```python
from build123d import *

# Parameters (mm, degrees)
CROQUIS1_W              = 74.8
CROQUIS1_H              = 11.8
SALIENTE_EXTRUIR1_DEPTH = 2.5
CORTAR_EXTRUIR1_REACH   = 4.5
CROQUIS2_R              = 1.6


with BuildPart() as part:
    # Croquis1 → Saliente-Extruir1 (new body)
    with BuildSketch(Plane.XY):
        with Locations((0, -76)):
            Rectangle(CROQUIS1_W, CROQUIS1_H)
    extrude(amount=SALIENTE_EXTRUIR1_DEPTH)

    # Croquis2 → Cortar-Extruir1 (cut, up to next)
    with BuildSketch(Plane.XY.offset(2.5), mode=Mode.PRIVATE) as cortar_extruir1_sk1:
        with Locations((-22.5, -76)):
            Circle(CROQUIS2_R)
    cortar_extruir1_tool1 = extrude(cortar_extruir1_sk1.sketch, amount=-CORTAR_EXTRUIR1_REACH, mode=Mode.PRIVATE) & part.part
    add(cortar_extruir1_tool1.solids().sort_by_distance((-22.5, -76, 2.5))[0], mode=Mode.SUBTRACT)
    # Croquis2 → Cortar-Extruir1 (cut, up to next)
    with BuildSketch(Plane.XY.offset(2.5), mode=Mode.PRIVATE) as cortar_extruir1_sk2:
        with Locations((22.5, -76)):
            Circle(CROQUIS2_R)
    cortar_extruir1_tool2 = extrude(cortar_extruir1_sk2.sketch, amount=-CORTAR_EXTRUIR1_REACH, mode=Mode.PRIVATE) & part.part
    add(cortar_extruir1_tool2.solids().sort_by_distance((22.5, -76, 2.5))[0], mode=Mode.SUBTRACT)
    # Croquis2 → Cortar-Extruir1 (cut, up to next)
    with BuildSketch(Plane.XY.offset(2.5), mode=Mode.PRIVATE) as cortar_extruir1_sk3:
        with Locations((-7.5, -76)):
            Circle(CROQUIS2_R)
    cortar_extruir1_tool3 = extrude(cortar_extruir1_sk3.sketch, amount=-CORTAR_EXTRUIR1_REACH, mode=Mode.PRIVATE) & part.part
    add(cortar_extruir1_tool3.solids().sort_by_distance((-7.5, -76, 2.5))[0], mode=Mode.SUBTRACT)
    # Croquis2 → Cortar-Extruir1 (cut, up to next)
    with BuildSketch(Plane.XY.offset(2.5), mode=Mode.PRIVATE) as cortar_extruir1_sk4:
        with Locations((7.5, -76)):
            Circle(CROQUIS2_R)
    cortar_extruir1_tool4 = extrude(cortar_extruir1_sk4.sketch, amount=-CORTAR_EXTRUIR1_REACH, mode=Mode.PRIVATE) & part.part
    add(cortar_extruir1_tool4.solids().sort_by_distance((7.5, -76, 2.5))[0], mode=Mode.SUBTRACT)


solid = part.part
```
CAD build for the part. Positions are in the model's coordinates, mm. Give positions to 0.01 mm unless a question says otherwise; leave off trailing zeros. Order: outer loops, then holes, each group sorted by start corner. A loop starts at its lowest first (then second) coordinate and runs counter-clockwise, first axis right, second up.
(1) Saw through at C-C, the plane z = 0.4. Give the cut face in (x, y), then the cut area to 3 significant figures.
(2) Saw through at A-A, the plane y = -76. Give the cut face in (x, z).
(3) Mould opens along Y. For faces 1 (the flat face through (-1, -76, 2.5)), 2 (the flat face through (-1, -81.9, 1)), 3 (the cylindrical face through (-7.708, -74.414, 1.268)) say: released by +Y, released by -Y, zero draft, split by the parting line, or undercut.
(4) Saw through at B-B, the plane x = -7.5. Give the cut face in (y, z).
(5) Drill centre lines: L1, parallel to X at y = -76, z = 0.5; L2, parallel to Y at x = 22.5, z = 0.9; L3, parallel to X at y = -77, z = 0.7. Where is each one in solid material? Low to high.
Results found:
1. outline: (-37.4, -81.9) - (37.4, -81.9) - (37.4, -70.1) - (-37.4, -70.1) - close; hole circle Ø3.2 at (-22.5, -76); hole circle Ø3.2 at (-7.5, -76); hole circle Ø3.2 at (7.5, -76); hole circle Ø3.2 at (22.5, -76)
1. area: 850 mm2
2. outline: (-37.4, 0) - (-24.1, 0) - (-24.1, 2.5) - (-37.4, 2.5) - close; (-20.9, 0) - (-9.1, 0) - (-9.1, 2.5) - (-20.9, 2.5) - close; (-5.9, 0) - (5.9, 0) - (5.9, 2.5) - (-5.9, 2.5) - close; (9.1, 0) - (20.9, 0) - (20.9, 2.5) - (9.1, 2.5) - close; (24.1, 0) - (37.4, 0) - (37.4, 2.5) - (24.1, 2.5) - close
3. face 1: zero draft
3. face 2: released by -Y
3. face 3: undercut
4. outline: (-81.9, 0) - (-77.6, 0) - (-77.6, 2.5) - (-81.9, 2.5) - close; (-74.4, 0) - (-70.1, 0) - (-70.1, 2.5) - (-74.4, 2.5) - close
5. L1: x = -37.4 to -24.1, -20.9 to -9.1, -5.9 to 5.9, 9.1 to 20.9, 24.1 to 37.4
5. L2: y = -81.9 to -77.6, -74.4 to -70.1
5. L3: x = -37.4 to -23.75, -21.25 to -8.75, -6.25 to 6.25, 8.75 to 21.25, 23.75 to 37.4
